Design review of the part built by this model. Coordinates are the model's own, in mm. Give positions to 0.01 mm unless a question says otherwise; leave off trailing zeros. Order: outer loops, then holes, each group sorted by start corner. A loop starts at its lowest first (then second) coordinate and runs counter-clockwise, first axis right, second up. Notation, with made-up numbers: (-2.5, -30) -> (25.5, -30) arc R32 cw to (25.5, -3) -> close; hole circle Ø6 at (-13.5, 28). An arc over 180 degrees is marked (long way). One line per item, written item: value. Start each with the question number.
1) Consider section D-D (z = -18). State the section outline as (x, y) points (3 decimals).
2) Consider section A-A (z = -9). State the section outline as (x, y) points (3 decimals).
3) Consider section C-C (y = -2.5). State the section outline as (x, z) points.
4) The part is to be moulded in two halves that separate along X. For faces 1 (the face through (1.48, 10.85, 22.45)), 2 (the face through (9.9, 22, 18.2)), 3 (the face through (-4.444, 11.86, -20.013)), say which applies: released by +X, released by -X, zero draft, split by the parting line, or undercut.
5) Consider section B-B (y = 5). State the section outline as (x, z) points, plus the area to 3 significant figures.
6) For pin 1 (4 mm diameter, centred on x = -2, z = -10.5, fed in from +Y); pin 2 (8 mm diameter, centred on x = 14, y = 14.5, fed in from -Z); pin 3 (10 mm diameter, centred on y = 9, z = -13, fed in from -X), all flat-tipped, find the tip position at first contact; note any pin that passes through.
7) Wall thickness on line 1 along X through (y, z) = (12.75, 0); line 2 along Z through (x, y) = (3, 11.25): over which ranges is each line inside the solid? List them lowest first. Write a range as from..to.
Autodesk Inventor part; units mm, degrees
ref_plane "YZ Plane" through (0, 0, 0) normal (1, 0, 0) x (0, 1, 0)
ref_plane "XZ Plane" through (0, 0, 0) normal (0, 1, 0) x (-1, 0, 0)
ref_plane "XY Plane" through (0, 0, 0) normal (0, 0, 1) x (1, 0, 0)
sketch "Sketch1" plane through (0, 0, 0) normal (0, 1, 0) x (-1, 0, 0)
  circle A0 centre (0, 0) radius 22.5
  dimension "d0" = 45
extrude "Extrusion1" add sketch "Sketch1" along normal blind 2
sketch "Sketch2" plane through (0, 2, 0) normal (0, 1, 0) x (1, 0, 0)
  circle A0 centre (0, 0) radius 22.5
  circle A1 centre (0, 0) radius 22.5
  circle A2 centre (0, 0) radius 20.5
  dimension "d3" = 2
extrude "Extrusion2" add sketch "Sketch2" along normal blind 20
sketch "Sketch3" plane through (0, 0, 0) normal (0, 0, 1) x (1, 0, 0)
  line L0 (22.5, 0) -> (-22.5, 0)
  line L1 (22.5, 0) -> (0, 0)
  line L2 (0, 0) -> (0, -5)
  arc A0 (-22.5, 0) -> (0, -5) centre (0, 48.125) ccw
  dimension "d6" = 5
revolve "Revolution1" add sketch "Sketch3" angle 360 about axis through (0, 0, 0) along (0, -1, 0)
properties part number "Pieza 1.1 final" material "ABS Plastic"
Checked values:
1. outline: (-13.5, 0) arc R49.983 ccw to (13.5, 0) -> (13.5, 22) -> (9.811, 22) -> (9.811, 2) -> (-9.811, 2) -> (-9.811, 22) -> (-13.5, 22) -> close
2. outline: (-20.622, 0) arc R52.357 ccw to (20.622, 0) -> (20.622, 22) -> (18.419, 22) -> (18.419, 2) -> (-18.419, 2) -> (-18.419, 22) -> (-20.622, 22) -> close
3. outline: circle Ø32.21 at (0, 0)
4. face 1: split by the parting line
4. face 2: zero draft
4. face 3: undercut
5. outline: circle Ø45 at (0, 0); hole circle Ø41 at (0, 0)
5. area: 270 mm^2
6. pin 1: stops at y = 2
6. pin 2: stops at z = -20.16
6. pin 3: stops at x = -21.03
7. line 1: x = -22.5..-20.5, 20.5..22.5
7. line 2: z = -22.3..-20.28, 20.28..22.3
